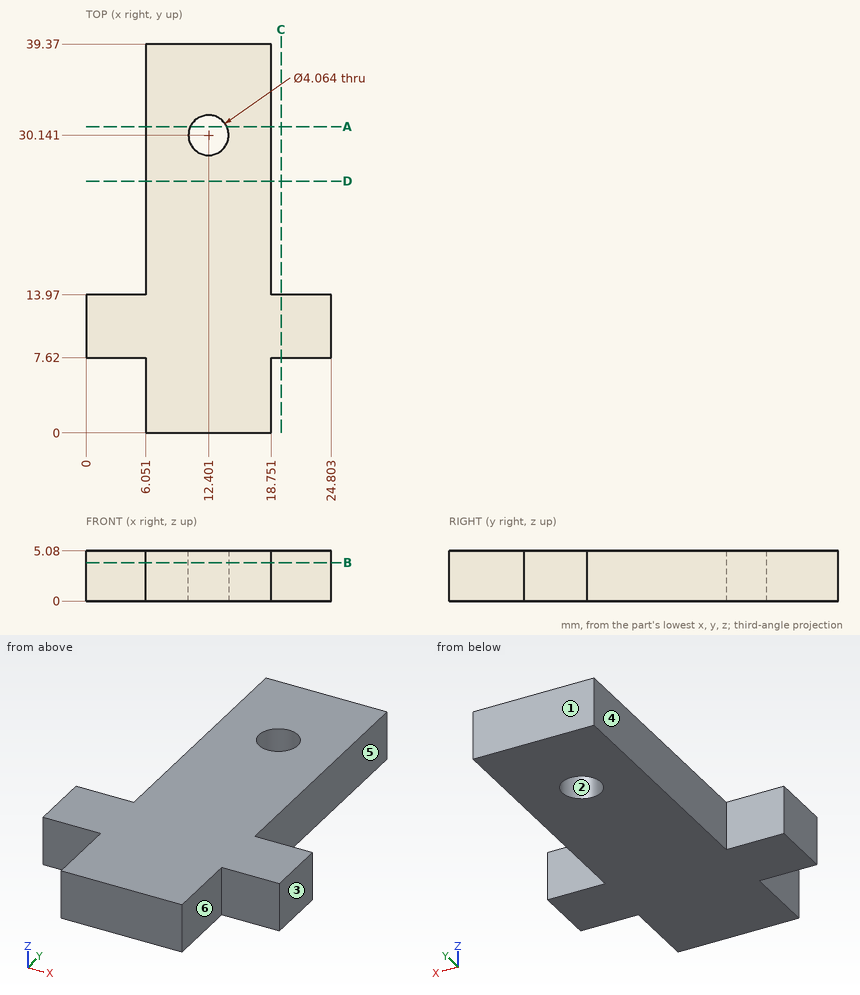
Design review of the part shown in the three views and the two pictorial views. Dimensions are in mm from the part's minimum x, y and z. A direction names the side the tool comes from. Give positions to 0.01 mm unless a question says otherwise; leave off trailing zeros. Write each loop counter-clockwise with the first axis right and the second up, starting at its lowest first coordinate (ties: lowest second). Pieces come first, ordered by that corner, then holes.
Item 1: Take a section at D-D (y = 25.5). Give the boundary of the cut face in (x, z), and give its area (3 significant figures).
Item 2: Take a section at C-C (x = 19.75). Give the boundary of the cut face in (y, z).
Item 3: Take a section at A-A (y = 31). Give the boundary of the cut face in (x, z), and give its area (3 significant figures).
Item 4: Wall thickness on probe 1 along X at (y, z) = (3.5, 2.35); probe 2 along X at (y, z) = (29, 0.25); probe 3 along Y at (x, z) = (11, 4.2): over which ranges is each line inside the solid? List them lowest first.
Item 5: The part is to be moulded in two halves that separate along Y. For the marked faces 1, 2 and 3, say which applies: +Y half, -Y half, draft (parallel to the pull), parting line (faces both ways), or undercut.
Item 6: Machinability: for the marked faces 4, 5 and 6, which of the approach directions +Z, -Z, +X, -X, +Y, -Y give a long, thin tool a straight path to every point of the face, cutting with its end or side? Answer none if there is none.
Item 7: Take a section at B-B (z = 3.9). Give the boundary of the cut face in (x, y).
Established:
1. outline: (6.05, 0) - (18.75, 0) - (18.75, 5.08) - (6.05, 5.08) - close
1. area: 64.5 mm2
2. outline: (7.62, 0) - (13.97, 0) - (13.97, 5.08) - (7.62, 5.08) - close
3. outline: (6.05, 0) - (10.56, 0) - (10.56, 5.08) - (6.05, 5.08) - close; (14.24, 0) - (18.75, 0) - (18.75, 5.08) - (14.24, 5.08) - close
3. area: 45.8 mm2
4. probe 1: x = 6.05 to 18.75
4. probe 2: x = 6.05 to 10.72, 14.08 to 18.75
4. probe 3: y = 0 to 28.67, 31.61 to 39.37
5. face 1: +Y half
5. face 2: undercut
5. face 3: draft
6. face 4: +Z, -Z, -X, +Y
6. face 5: +Z, -Z, +X, +Y
6. face 6: +Z, -Z, +X, -Y
7. outline: (0, 7.62) - (6.05, 7.62) - (6.05, 0) - (18.75, 0) - (18.75, 7.62) - (24.8, 7.62) - (24.8, 13.97) - (18.75, 13.97) - (18.75, 39.37) - (6.05, 39.37) - (6.05, 13.97) - (0, 13.97) - close; hole circle Ø4.06 at (12.4, 30.14)
